Verification items for this drawing (mm, ordinates from the low corner). A direction names the side the tool comes from. Give positions to 0.01 mm unless a question says otherwise; leave off trailing zeros. Loops run counter-clockwise (first coordinate to the right, second up) from the corner with the lowest first, then second, coordinate; pieces in that order, holes last. Notation, with made-up numbers: (-16, 17.5) -> (12, 17.5) arc R20 ccw to (12, 25.5) -> close; hole circle Ø1 at (-8.75, 32.25). An arc over 180 degrees is marked (long way). Answer in a Markdown table with one row per item. Add a question column.
Q1. Section check D-D on y = 43.5. Enter the section's corners in (x, z).
Q2. Section check C-C on z = 12.5. Enter the section's corners in (x, y), and give its area (3 significant figures).
Q3. Gauge pin test, flat ends, axial feed: P1, Ø1.5, axis at y = 47.5, z = 19, coming from the +X side; P2, Ø10, axis at y = 42.5, z = 6, coming from the -X side; P3, Ø2, axis at x = 12.5, y = 21, coming from the +Z side. Record the tip position at first contact, or that the pin passes through.
Q4. Set-up check for the marked faces 1 and 2: record each of +Z, -Z, +X, -X, +Y, -Y from which the full face is reachable in a straight line by a thin tool's end or side.
Q5. Material ranges on probe 1 along Y at (x, z) = (19, 19); probe 2 along X at (y, z) = (32.5, 13); probe 3 along X at (y, z) = (13, 7.5), recorded low to high.
Q6. Section check B-B on x = 12.5. Enter the section's corners in (y, z).
Q7. Section check A-A on z = 2.5. Enter the section's corners in (x, y), and give its area (3 significant figures).
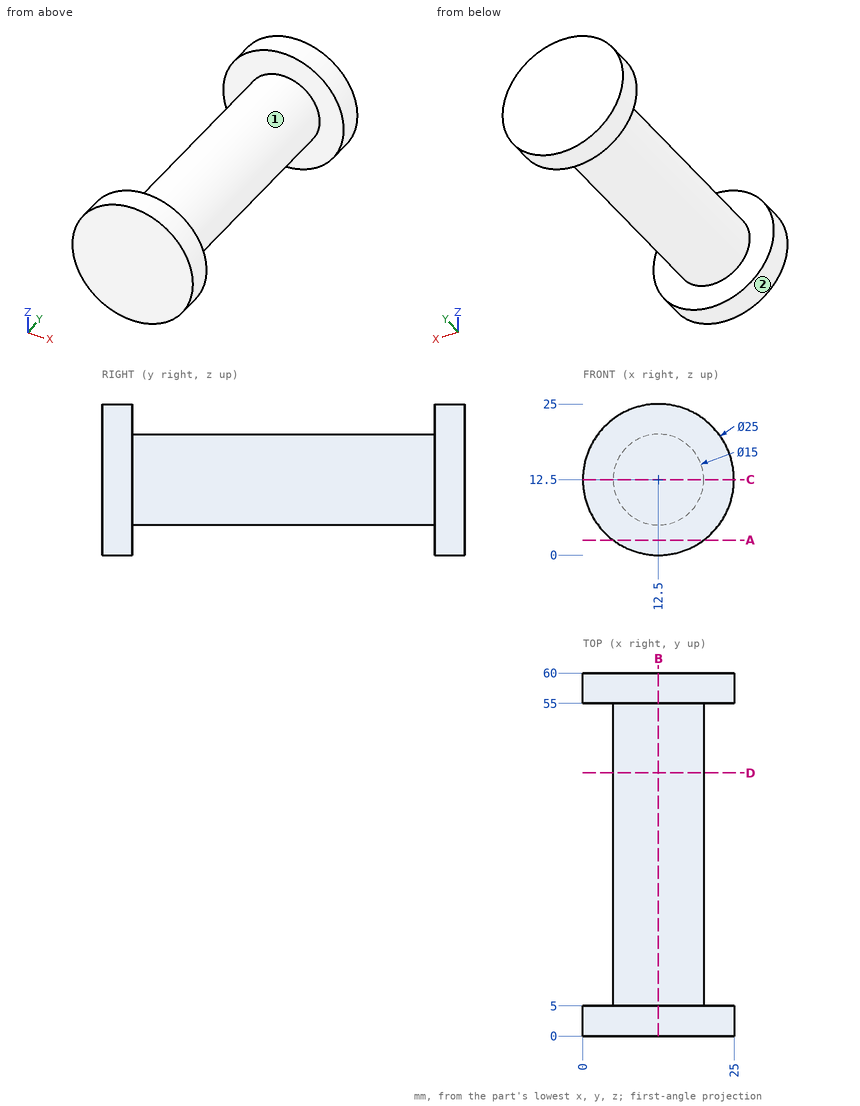
Taken from the geometry:
| question | item | result |
|---|---|---|
| 1 | outline | circle Ø15 at (12.5, 12.5) |
| 2 | outline | (0, 0) -> (25, 0) -> (25, 5) -> (20, 5) -> (20, 55) -> (25, 55) -> (25, 60) -> (0, 60) -> (0, 55) -> (5, 55) -> (5, 5) -> (0, 5) -> close |
| 2 | area | 1,000 mm² |
| 3 | P1 | stops at x = 17.32 |
| 3 | P2 | stops at x = 5.15 |
| 3 | P3 | stops at z = 20 |
| 4 | face 1 | none |
| 4 | face 2 | +Y, -Y |
| 5 | probe 1 | y = 0 to 5, 55 to 60 |
| 5 | probe 2 | x = 5.02 to 19.98 |
| 5 | probe 3 | x = 6.91 to 18.09 |
| 6 | outline | (0, 0) -> (5, 0) -> (5, 5) -> (55, 5) -> (55, 0) -> (60, 0) -> (60, 25) -> (55, 25) -> (55, 20) -> (5, 20) -> (5, 25) -> (0, 25) -> close |
| 7 | outline | (5, 0) -> (20, 0) -> (20, 5) -> (5, 5) -> close; (5, 55) -> (20, 55) -> (20, 60) -> (5, 60) -> close |
| 7 | area | 150 mm² |
